Could you check a few things on this model? Use its own coordinates, in mm. A direction names the side the tool comes from. Coordinates: 2 decimals unless noted, no trailing zeros. Loops run counter-clockwise (first coordinate to the right, second up) from the corner with the lowest first, then second, coordinate; pieces in that order, holes last. Notation, with made-up numbers: (58, 55) -> (76, 55) arc R12 ccw to (76, 59) -> close; hole circle Ø3 at (30, -37.5). An arc over 180 degrees is marked (long way). One line per question, with ' | ' between items.
Autodesk Inventor part; units mm, degrees
ref_plane "YZ Plane" through (0, 0, 0) normal (1, 0, 0) x (0, 1, 0)
ref_plane "XZ Plane" through (0, 0, 0) normal (0, 1, 0) x (-1, 0, 0)
ref_plane "XY Plane" through (0, 0, 0) normal (0, 0, 1) x (1, 0, 0)
sketch "Sketch1" plane through (0, 0, 0) normal (0, 1, 0) x (-1, 0, 0)
  line L0 (3.6632, 6.4956) -> (-8.8368, 6.4956)
  line L1 (-8.8368, 6.4956) -> (-8.8368, -10.5044)
  line L2 (-8.8368, -10.5044) -> (3.6632, -10.5044)
  line L3 (3.6632, -10.5044) -> (3.6632, 6.4956)
  line L4 (0.9132, -10.5044) -> (-6.0868, -10.5044)
  point P0 (0, 0)
  dimension "d0" = 17
  dimension "d1" = 12.5
extrude "Extrusion1" add sketch "Sketch1" along normal blind 7
chamfer "Chamfer1" distance 3 angle 45 1 edges at (2.5868, 0, 6.4956)
sketch "Sketch2" plane through (0, 7, 0) normal (0, 1, 0) x (1, 0, 0)
  circle A0 centre (2.5868, 3.1044) radius 5.025
  line L0 (8.8368, -6.4956) -> (8.8368, 10.5044)
  line L1 (-3.6632, -6.4956) -> (8.8368, -6.4956)
  point P0 (0, 0)
  dimension "d7" = 10.05
  dimension "d8" = 6.25
  dimension "d9" = 9.6
extrude "Extrusion2" cut sketch "Sketch2" against normal up to next
sketch "Sketch3" plane through (0, 7, 0) normal (0, 1, 0) x (1, 0, 0)
  line L0 (-3.6632, -6.4956) -> (8.8368, -6.4956)
  line L1 (1.5868, -6.4956) -> (3.5868, -6.4956)
  line L2 (3.5868, -6.4956) -> (3.5868, 0)
  line L3 (3.5868, 0) -> (1.5868, 0)
  line L4 (1.5868, 0) -> (1.5868, -6.4956)
  line L5 (8.8368, -6.4956) -> (8.8368, 10.5044)
  line L6 (-3.6632, 10.5044) -> (-3.6632, -6.4956)
  point P0 (0, 0)
  dimension "d16" = 2
  dimension "d17" = 12.5
  dimension "d18" = 5.25
extrude "Extrusion3" cut sketch "Sketch3" against normal through all
sketch "Sketch4" plane through (8.8368, 0, -10.5044) normal (1, 0, 0) x (0, 0, -1)
  line L0 (-17, 3) -> (-17, 7)
  line L1 (-17, 7) -> (0, 7)
  point P0 (-10.5044, 0)
  point P1 (-14.5, 4.5)
  dimension "d26" = 2.5
  dimension "d27" = 2.5
hole "Hole1" at (8.8368, 4.5, 3.9956) direction (-1, 0, 0) diameter 3.4 depth 5.25
sketch "Sketch5" plane through (1.5868, 7, 6.4956) normal (1, 0, 0) x (0, 0, -1)
  line L0 (0, 0) -> (17, 0)
  line L1 (0, -4) -> (0, 0)
  point P0 (6.4956, -7)
  point P1 (2.5, -2.5)
  dimension "d35" = 2.5
  dimension "d36" = 2.5
hole "Hole2" at (1.5868, 4.5, 3.9956) direction (-1, 0, 0) diameter 2.459 depth 5.25
sketch "Sketch6" plane through (8.8368, 0, -10.5044) normal (0, 0, -1) x (-1, 0, 0)
  line L0 (5.25, 7) -> (0, 7)
  line L1 (3.25, 7) -> (9.25, 7)
  line L2 (9.25, 7) -> (9.25, 0)
  line L3 (9.25, 0) -> (3.25, 0)
  line L4 (3.25, 0) -> (3.25, 7)
  line L5 (0, 0) -> (0, 7)
  point P0 (8.8368, 0)
  dimension "d40" = 6
  dimension "d41" = 7
  dimension "d42" = 3.25
extrude "Extrusion4" add sketch "Sketch6" along normal blind 10.85
fillet "Fillet1" radius 2 1 edges at (8.8368, 3.5, -10.5044)
fillet "Fillet2" radius 2 1 edges at (5.5868, 3.5, -10.5044)
fillet "Fillet3" radius 2 2 edges at (-3.6632, 3.5, -10.5044) (-0.4132, 3.5, -10.5044)
sketch "Sketch7" plane through (0, 7, 0) normal (0, 1, 0) x (1, 0, 0)
  point P0 (0, 0)
sketch "Sketch8" plane through (8.8368, 0, -21.3544) normal (0, 0, -1) x (-1, 0, 0)
  point P0 (8.8368, 0)
sketch "Sketch9" plane through (0, 7, 0) normal (0, 1, 0) x (1, 0, 0)
  line L0 (5.5868, 21.3544) -> (-0.4132, 21.3544)
  line L1 (5.5868, 21.3544) -> (8.5868, 24.3544)
  line L2 (8.5868, 24.3544) -> (8.5868, 30.3544)
  line L3 (-3.4132, 30.3544) -> (-3.4132, 24.3544)
  line L4 (-3.4132, 24.3544) -> (-0.4132, 21.3544)
  line L5 (8.5868, 30.3544) -> (5.5868, 33.3544)
  line L6 (5.5868, 33.3544) -> (-0.4132, 33.3544)
  line L7 (-0.4132, 33.3544) -> (-3.4132, 30.3544)
  line L8 (5.5868, 12.4335) -> (5.5868, 21.3544)
  line L9 (-0.4132, 12.4335) -> (-0.4132, 21.3544)
  point P0 (0, 0)
  dimension "d110" = 6
  dimension "d111" = 6
  dimension "d112" = 6
  dimension "d113" = 6
  dimension "d114" = 45
  dimension "d115" = 135
  dimension "d116" = 45
  dimension "d117" = 45
  dimension "d118" = 45
  dimension "d119" = 3
  dimension "d120" = 3
extrude "Extrusion5" add sketch "Sketch9" against normal blind 7
sketch "Sketch10" plane through (0, 7, 0) normal (0, 1, 0) x (1, 0, 0)
  circle A0 centre (2.5868, 27.3544) radius 3.25
  line L0 (5.5868, 33.3544) -> (-0.4132, 33.3544)
  line L1 (8.5868, 24.3544) -> (8.5868, 30.3544)
  line L2 (-3.4132, 30.3544) -> (-3.4132, 24.3544)
  point P0 (0, 0)
  dimension "d76" = 6.5
  dimension "d77" = 6
  dimension "d78" = 6
  dimension "d121" = 12
extrude "Extrusion6" cut sketch "Sketch10" against normal up to next
sketch "Sketch11" plane through (8.8368, 3, 6.4956) normal (1, 0, 0) x (0, 0, -1)
  point P0 (6.4956, -3)
sketch "Sketch12" plane through (5.8368, 0, -21.6044) normal (0.7071, 0, 0.7071) x (0.7071, 0, -0.7071)
  line L0 (-0.3536, 7) -> (3.8891, 7)
  line L1 (3.8891, 7) -> (3.8891, 0)
  point P0 (-19.4039, 0)
  dimension "d122" = 7
  dimension "d123" = 4.2426
hole "Hole3" [suppressed]
sketch "Sketch13" plane through (8.5868, 0, -30.3544) normal (0.7071, 0, -0.7071) x (-0.7071, 0, -0.7071)
  line L0 (4.2426, 7) -> (4.2426, 0)
  line L1 (4.2426, 0) -> (0, 0)
  point P0 (-15.392, 0)
hole "Hole4" [suppressed]
equation "\"d18\" = 0.5 * d17 - 0.5 * d16"
equation "\"d111\" = d110"
equation "\"d112\" = d110"
equation "\"d113\" = d110"
equation "\"d116\" = d114"
equation "\"d117\" = d116"
equation "\"d118\" = d117"
equation "\"d120\" = d119"
equation "\"d77\" = d78"
equation "\"d78\" = 0.5 * d121"
properties part number "dovetail stabilizer"
1) If we section it at A-A on x = 1: Please give me the cut outline in (y, z).
Data:
outline: (0, -33.35) -> (7, -33.35) -> (7, -30.19) -> (0, -30.19) -> close; (0, -24.52) -> (7, -24.52) -> (7, -7.87) -> (0, -7.87) -> close; (0, 1.66) -> (7, 1.66) -> (7, 6.5) -> (3, 6.5) -> (0, 3.5) -> close; hole circle Ø2.46 at (4.5, 4)
2) I'm going to push flat-ended pins straight in: pin 1 Ø1.4 at (y, z) = (4, 3.5) entering from -X; pin 2 Ø1 at (x, y) = (4.5, 1.5) entering from +Z; pin 3 Ø1.8 at (y, z) = (4, -28.5) entering from -X; pin 4 Ø1.8 at (y, z) = (5, -27) entering from +X. Where does each tip first touch, or does it pass through?
Data:
pin 1: x = -3.66 | pin 2: z = 5.5 | pin 3: x = -3.41 | pin 4: x = 8.59
3) On a 3-axis mill with a long thin cutter (end or side, diameter ignored), from which of +Z, -Z, +X, -X, +Y, -Y can I reach the whole of each face in a straight line? I mean faces 5 (the face through (5.587, 3, -17)), 6 (the face through (3.587, 2.77, 4.71)), 7 (the face through (2.794, 3.549, -8.125)), 8 (the face through (-1.934, 3.549, -22.875)). Say none if no direction works.
Data:
face 5: +X, +Y, -Y | face 6: +Z, +Y, -Y | face 7: +Y, -Y | face 8: -X, +Y, -Y
4) If we section it at D-D on y = 4.5: Give the number of separate pieces and of enclosed holes in the cut face, and give its area (3 significant figures).
Data:
separate pieces: 3 | enclosed holes: 1 | area: 251 mm²
5) If we section it at B-B on z = -4: Please give me the cut outline in (x, y).
Data:
outline: (-3.66, 0) -> (-2.36, 0) -> (-2.36, 7) -> (-3.66, 7) -> close; (7.53, 0) -> (8.84, 0) -> (8.84, 7) -> (7.53, 7) -> close
6) I need wall thicknesses on line 1 along Z through (x, y) = (0, 6.75); line 2 along Z through (x, y) = (1, 2.75); line 3 along X through (y, z) = (2, 3). Which ranges of each line are inside material? Lowest first, please. Write a range as from..to.
Data:
line 1: -33.35..-29.32, -25.39..-7.41, 1.2..6.5 | line 2: -33.35..-30.19, -24.52..-7.87, 1.66..6.25 | line 3: -3.66..1.59, 3.59..8.84
7) We'd pull the mould along Y, two halves only. Please class faces 1 (the face through (-1.07, 5.25, 4.97)), 2 (the face through (2, 7, -14)), 3 (the face through (6.175, 6.008, 3.211)), 4 (the face through (-3.192, 3.549, -9.794)): pulls with the +Y half, pulls with the -Y half, needs draft (parallel to the pull), parting line crosses it, or undercut.
Data:
face 1: undercut | face 2: pulls with the +Y half | face 3: undercut | face 4: needs draft
8) If we section it at C-C on x = 2.5: Please give me the cut outline in (y, z), and give its area (3 significant figures).
Data:
outline: (0, -33.35) -> (7, -33.35) -> (7, -30.6) -> (0, -30.6) -> close; (0, -24.11) -> (7, -24.11) -> (7, -8.13) -> (0, -8.13) -> close | area: 131 mm²
